Part model, mm, in its own coordinate system. A direction names the side the tool comes from. Give positions to 0.01 mm unless a question says otherwise; leave off trailing zeros. Write each loop counter-clockwise with the first axis right and the second up, starting at its lowest first coordinate (ties: lowest second). Pieces come first, ordered by that corner, then holes.
```python
from build123d import *

# Parameters (mm, degrees)
SKETCH1_R                              = 2.5
BOSS_EXTRUDE1_DEPTH                    = 1
FILLET1_R                              = 0.25
SKETCH2_R                              = 1.5
BOSS_EXTRUDE2_DEPTH                    = 3
F_1_16_0_07874016_DIAMETER_HOLE1_D     = 2.000000064
F_1_16_0_07874016_DIAMETER_HOLE1_DEPTH = 1.75
F_1_16_0_07874016_DIAMETER_HOLE1_TIP   = 0.600860638
FILLET2_R                              = 0.15


with BuildPart() as part:
    # Sketch1 → Boss-Extrude1 (new body)
    with BuildSketch(Plane(origin=(0, 0, 0), x_dir=(1, 0, 0), z_dir=(0, 1, 0))):
        with Locations(Location((0, 0, 0), (0, 0, 270))):
            Circle(SKETCH1_R)
    extrude(amount=BOSS_EXTRUDE1_DEPTH)

    # Fillet1
    fillet1_edges = [part.edges().sort_by_distance(p)[0] for p in [
        (0, 0, -2.5),
        (0, 1, -2.5),
    ]]
    fillet(fillet1_edges, radius=FILLET1_R)

    # Sketch2 → Boss-Extrude2 (add)
    with BuildSketch(Plane.XZ):
        with Locations(Location((0, 0, 0), (0, 0, 90))):
            Circle(SKETCH2_R)
    extrude(amount=BOSS_EXTRUDE2_DEPTH)

    # 1/16 (0.07874016) Diameter Hole1
    with Locations(Plane(origin=(0, -3, 0), x_dir=(-1, 0, 0), z_dir=(0, -1, 0))):
        with Locations((0, 0)):
            Hole(F_1_16_0_07874016_DIAMETER_HOLE1_D / 2, depth=F_1_16_0_07874016_DIAMETER_HOLE1_DEPTH)
            with Locations((0, 0, -(F_1_16_0_07874016_DIAMETER_HOLE1_DEPTH + F_1_16_0_07874016_DIAMETER_HOLE1_TIP / 2))):  # 118° drill point
                Cone(0, F_1_16_0_07874016_DIAMETER_HOLE1_D / 2, F_1_16_0_07874016_DIAMETER_HOLE1_TIP, mode=Mode.SUBTRACT)

    # Fillet2
    fillet2_edges = [part.edges().sort_by_distance(p)[0] for p in [
        (-1.000000032, -3, 0),
    ]]
    fillet(fillet2_edges, radius=FILLET2_R)


solid = part.part
```
1) Wall check: L1, parallel to X at y = -2.1, z = 0; L2, parallel to Y at x = 0.2, z = -2.25; L3, parallel to X at y = -2.6, z = -0.6. Give the ranges that are in metal, low to high.
Answers follow:
L1: x = -1.5 to -1, 1 to 1.5
L2: y = 0 to 1
L3: x = -1.37 to -0.8, 0.8 to 1.37
2) Two-plate mould, pull along Z, no slides. Class faces 1 (the face through (1, -2, 0)), 2 (the face through (0, 0, -2)), 3 (the face through (-2.44, 0.5, -0.54)): +Z half, -Z half, draft (parallel to the pull), parting line (faces both ways), or undercut.
Answers follow:
face 1: undercut
face 2: draft
face 3: parting line
3) Saw through at B-B, the plane y = -0.45. Write the cut outline in (x, z).
Answers follow:
outline: circle Ø3 at (0, 0)
4) Saw through at A-A, the plane y = -2.05. Write the cut outline in (x, z).
Answers follow:
outline: circle Ø3 at (0, 0); hole circle Ø2 at (0, 0)
5) 3-axis set-ups, long thin cutter, end or side, ignore diameter. For faces 4 (the face through (-0.45, -1.48, 1.43)), 5 (the face through (0, 1, 0)): which of +Z, -Z, +X, -X, +Y, -Y reach the whole face in a straight line?
Answers follow:
face 4: -Y
face 5: +Z, -Z, +X, -X, +Y
6) Pin check, flat tips, straight feed: pin 1 Ø1.5 at (y, z) = (-2, -1.5) entering from +X; pin 2 Ø2 at (y, z) = (-2, -0.5) entering from +X; pin 3 Ø1.5 at (x, y) = (1.5, -1.5) entering from -Z. Stop position of each tip, or through.
Answers follow:
pin 1: stops at x = 1.3
pin 2: stops at x = 1.5
pin 3: stops at z = -1.3
